Design review of the part built by this model. Coordinates are the model's own, in mm. Face numbers are marked on the shaded views. A direction names the side the tool comes from. Give positions to 0.01 mm unless a question says otherwise; leave off trailing zeros. Loops run counter-clockwise (first coordinate to the right, second up) from the corner with the lowest first, then second, coordinate; pieces in that order, holes last. Notation, with made-up numbers: M 1,36.5 L 6,36.5 A20 ccw 6,67.5 Z; hole C 43.25,67 d4. An arc over 180 degrees is marked long. Use a Markdown table: item, result. Add a question column.
(1) Add section B-B, the plane x = 45. Give the boundary of the cut face in (y, z).
(2) Add section D-D, the plane z = -60. Give the boundary of the cut face in (x, y).
(3) For the marked faces 5, 6, 7 and 8, list the 3-axis set-ups (+Z, -Z, +X, -X, +Y, -Y) from which the entire face can be reached by the end or side of a thin tool; tool diameter is ignored.
(4) Add section A-A, the plane y = 37. Give the boundary of the cut face in (x, z).
(5) For probe 1 along Z at (x, y) = (-4.5, 33.5); probe 2 along X at (y, z) = (46, -60); probe 3 along X at (y, z) = (28.5, -39), list the stretches that pass through material, from the lowest coordinate up.
(6) Draft analysis for pull direction X (two halves, no side actions). For the marked faces 1, 2, 3 and 4, state which applies: pulls with the +X half, pulls with the -X half, needs draft (parallel to the pull), parting line crosses it, or undercut.
(7) Add section C-C, the plane z = -14.5. Give the boundary of the cut face in (x, y).
(8) Insertion check: pin 1 Ø6.5 at (x, y) = (-5, 41) entering from -Z; pin 2 Ø5 at (x, y) = (20, 60) entering from +Z; pin 3 Ø5 at (x, z) = (21, -50.5) entering from -Y. Each pin has a flat end and moves straight along its axis. Give the tip position at first contact, or say it passes through.
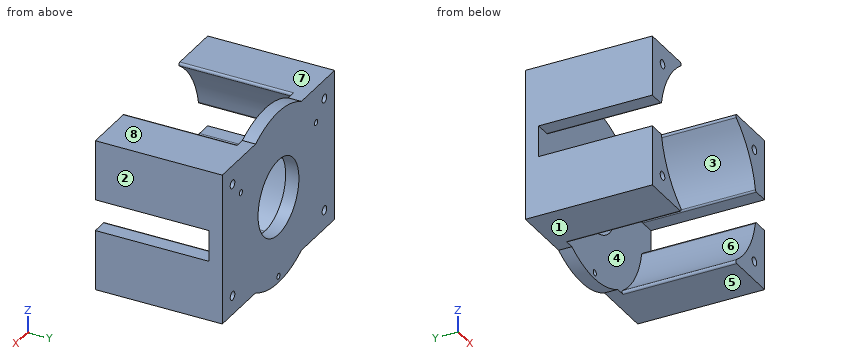
```python
from build123d import *

# Parameters (mm, degrees)
SKETCH1_R             = 2.25
BOSS_EXTRUDE1_DEPTH   = 60
BOSS_EXTRUDE1_2_DEPTH = 60
BOSS_EXTRUDE1_3_DEPTH = 60
BOSS_EXTRUDE1_4_DEPTH = 60
SKETCH5_R             = 1.5
SKETCH5_R_2           = 20
SKETCH5_R_3           = 2.25
BOSS_EXTRUDE3_DEPTH   = 7
FILLET1_R             = 1


with BuildPart() as part:
    # Sketch1 → Boss-Extrude1 (new body)
    with BuildSketch(Plane(origin=(0, 0, 0), x_dir=(1, 0, 0), z_dir=(0, 1, 0))):
        with BuildLine():
            ThreePointArc((20.608966812, 70), (6.336439637, 56.458488242), (-1.117716003, 38.250986042))
            Line((-1.117716003, 38.250986042), (-10, 38.250986042))
            Line((-10, 38.250986042), (-10, 70))
            Line((-10, 70), (20.608966812, 70))
        make_face()
        with Locations(Location((0, 60, 0), (0, 0, 270))):
            Circle(SKETCH1_R, mode=Mode.SUBTRACT)
    extrude(amount=BOSS_EXTRUDE1_DEPTH)



with BuildPart() as body_2:
    # Sketch1 → Boss-Extrude1 2 (new body)
    with BuildSketch(Plane(origin=(0, 0, 0), x_dir=(1, 0, 0), z_dir=(0, 1, 0))):
        with BuildLine():
            ThreePointArc((-1.117716003, 21.749013958), (6.336439637, 3.541511758), (20.608966812, -10))
            Line((20.608966812, -10), (-10, -10))
            Line((-10, -10), (-10, 21.749013958))
            Line((-10, 21.749013958), (-1.117716003, 21.749013958))
        make_face()
        with Locations(Location((0, 0, 0), (0, 0, 270))):
            Circle(SKETCH1_R, mode=Mode.SUBTRACT)
    extrude(amount=BOSS_EXTRUDE1_2_DEPTH)


with BuildPart() as body_3:
    # Sketch1 → Boss-Extrude1 3 (new body)
    with BuildSketch(Plane(origin=(0, 0, 0), x_dir=(1, 0, 0), z_dir=(0, 1, 0))):
        with BuildLine():
            ThreePointArc((91.117716003, 38.250986042), (83.663560363, 56.458488242), (69.391033188, 70))
            Line((69.391033188, 70), (100, 70))
            Line((100, 70), (100, 38.250986042))
            Line((100, 38.250986042), (91.117716003, 38.250986042))
        make_face()
        with Locations(Location((90, 60, 0), (0, 0, 270))):
            Circle(SKETCH1_R, mode=Mode.SUBTRACT)
    extrude(amount=BOSS_EXTRUDE1_3_DEPTH)


with BuildPart() as body_4:
    # Sketch1 → Boss-Extrude1 4 (new body)
    with BuildSketch(Plane(origin=(0, 0, 0), x_dir=(1, 0, 0), z_dir=(0, 1, 0))):
        with BuildLine():
            ThreePointArc((69.391033188, -10), (83.663560363, 3.541511758), (91.117716003, 21.749013958))
            Line((91.117716003, 21.749013958), (100, 21.749013958))
            Line((100, 21.749013958), (100, -10))
            Line((100, -10), (69.391033188, -10))
        make_face()
        with Locations(Location((90, 0, 0), (0, 0, 270))):
            Circle(SKETCH1_R, mode=Mode.SUBTRACT)
    extrude(amount=BOSS_EXTRUDE1_4_DEPTH)


with BuildPart() as part_1:
    add(part.part)

    add(body_2.part)  # Boss-Extrude3 merges body 2

    add(body_3.part)  # Boss-Extrude3 merges body 3

    add(body_4.part)  # Boss-Extrude3 merges body 4
    # Sketch5 → Boss-Extrude3 (add)
    with BuildSketch(Plane(origin=(0, 60, 0), x_dir=(1, 0, 0), z_dir=(0, 1, 0))):
        with BuildLine():
            Line((-10, 70), (22.589678717, 70))
            ThreePointArc((22.589678717, 70), (45, 75.85), (67.410321283, 70))
            Line((67.410321283, 70), (100, 70))
            Line((100, 70), (100, -10))
            Line((100, -10), (67.410321283, -10))
            ThreePointArc((67.410321283, -10), (45, -15.85), (22.589678717, -10))
            Line((22.589678717, -10), (-10, -10))
            Line((-10, -10), (-10, 70))
        make_face()
        with Locations(Location((81.806079661, 8.75, 0), (0, 0, 270))):
            Circle(SKETCH5_R, mode=Mode.SUBTRACT)
        with Locations(Location((45, 72.5, 0), (0, 0, 270))):
            Circle(SKETCH5_R, mode=Mode.SUBTRACT)
        with Locations(Location((8.193920339, 8.75, 0), (0, 0, 270))):
            Circle(SKETCH5_R, mode=Mode.SUBTRACT)
        with Locations(Location((45, 30, 0), (0, 0, 270))):
            Circle(SKETCH5_R_2, mode=Mode.SUBTRACT)
        with Locations(Location((90, 60, 0), (0, 0, 270))):
            Circle(SKETCH5_R_3, mode=Mode.SUBTRACT)
        with Locations(Location((90, 0, 0), (0, 0, 270))):
            Circle(SKETCH5_R_3, mode=Mode.SUBTRACT)
        with Locations(Location((0, 0, 0), (0, 0, 270))):
            Circle(SKETCH5_R_3, mode=Mode.SUBTRACT)
        with Locations(Location((0, 60, 0), (0, 0, 270))):
            Circle(SKETCH5_R_3, mode=Mode.SUBTRACT)
    extrude(amount=BOSS_EXTRUDE3_DEPTH)

    # Fillet1
    fillet1_edges = [part_1.edges().sort_by_distance(p)[0] for p in [
        (-1.117716003, 30, -38.250986042),
        (20.608966812, 30, -70),
        (20.608966812, 30, 10),
        (-1.117716003, 30, -21.749013958),
        (69.391033188, 30, -70),
        (91.117716003, 30, -38.250986042),
        (91.117716003, 30, -21.749013958),
        (69.391033188, 30, 10),
    ]]
    fillet(fillet1_edges, radius=FILLET1_R)


solid = part_1.part
```
Established:
| question | item | result |
|---|---|---|
| 1 | outline | M 60,-75.85 L 67,-75.85 L 67,-74 L 60,-74 Z; M 60,-71 L 67,-71 L 67,-50 L 60,-50 Z; M 60,-10 L 67,-10 L 67,15.85 L 60,15.85 Z |
| 2 | outline | M -10,0 L -2.25,0 L -2.25,67 L -10,67 Z; M 2.25,0 L 9.01,0 L 9.01,60 L 80.99,60 L 80.99,0 L 87.75,0 L 87.75,67 L 2.25,67 Z; M 92.25,0 L 100,0 L 100,67 L 92.25,67 Z |
| 3 | face 5 | -Z, +X, +Y, -Y |
| 3 | face 6 | -Y |
| 3 | face 7 | +Z, -X, +Y, -Y |
| 3 | face 8 | +Z, +X, +Y, -Y |
| 4 | outline | M -10,-70 L 17.28,-70 A1 ccw 17.86,-68.18 A46.85 cw -0.97,-39.06 A1 ccw -1.95,-38.25 L -10,-38.25 Z; M -10,-21.75 L -1.95,-21.75 A1 ccw -0.97,-20.94 A46.85 cw 17.86,8.18 A1 ccw 17.28,10 L -10,10 Z; M 72.14,-68.18 A1 ccw 72.72,-70 L 100,-70 L 100,-38.25 L 91.95,-38.25 A1 ccw 90.97,-39.06 A46.85 cw Z; M 72.14,8.18 A46.85 cw 90.97,-20.94 A1 ccw 91.95,-21.75 L 100,-21.75 L 100,10 L 72.72,10 A1 ccw Z; hole C 0,-60 d4.5; hole C 0,0 d4.5; hole C 90,-60 d4.5; hole C 90,0 d4.5 |
| 5 | probe 1 | -70 to -38.25, -21.75 to 10 |
| 5 | probe 2 | -10 to -2.25, 2.25 to 9.01, 80.99 to 87.75, 92.25 to 100 |
| 5 | probe 3 | -10 to -0.98, 90.98 to 100 |
| 6 | face 1 | needs draft |
| 6 | face 2 | pulls with the +X half |
| 6 | face 3 | undercut |
| 6 | face 4 | undercut |
| 7 | outline | M -10,0 L 0.79,0 L 0.79,60 L 32.36,60 L 32.36,67 L -10,67 Z; M 57.64,60 L 89.21,60 L 89.21,0 L 100,0 L 100,67 L 57.64,67 Z |
| 8 | pin 1 | z = -70 |
| 8 | pin 2 | z = 10 |
| 8 | pin 3 | y = 60 |
